from build123d import *

# Parameters (mm, degrees)
SKETCH_1_R      = 1.65
SKETCH_1_R_2    = 5
EXTRUDE_1_DEPTH = 3
FILLET_1_R      = 1


with BuildPart() as part:
    # 草图1 → 凸台-拉伸1 (new body)
    with BuildSketch(Plane.XY):
        with BuildLine():
            Line((-5.5, 2.397915762), (-8, -79.435617584))
            ThreePointArc((-8, -79.435617584), (0, -112.5), (8, -79.435617584))
            Line((8, -79.435617584), (5.5, 2.397915762))
            ThreePointArc((5.5, 2.397915762), (0, 6), (-5.5, 2.397915762))
        make_face()
        Circle(SKETCH_1_R, mode=Mode.SUBTRACT)
        with Locations((0, -95)):
            Circle(SKETCH_1_R_2, mode=Mode.SUBTRACT)
        with BuildLine():
            Line((-3.203324226, -2.80246125), (-3.504023082, -12.645361196))
            Line((-3.504023082, -12.645361196), (3.713679897, -12.645361196))
            Line((3.713679897, -12.645361196), (3.40536458, -2.553148492))
            ThreePointArc((3.40536458, -2.553148492), (0.16045027, -4.253155401), (-3.203324226, -2.80246125))
        make_face(mode=Mode.SUBTRACT)
        Polygon((-3.570265581, -14.813704302), (-3.957626018, -27.493333612), (4.167282834, -27.493333612), (3.779922396, -14.813704302), align=None, mode=Mode.SUBTRACT)
        Polygon((-4.048518432, -30.468552565), (4.258175248, -30.468552565), (4.818203506, -48.800189025), (-4.60854669, -48.800189025), align=None, mode=Mode.SUBTRACT)
        with BuildLine():
            Line((-4.696319338, -51.673287395), (-5.408181825, -74.974976421))
            ThreePointArc((-5.408181825, -74.974976421), (0.132605518, -74.257955362), (5.66377239, -75.045760292))
            Line((5.66377239, -75.045760292), (4.949747468, -51.673287395))
            Line((4.949747468, -51.673287395), (-4.696319338, -51.673287395))
        make_face(mode=Mode.SUBTRACT)
        with BuildLine():
            Line((0, -81), (0, -88))
            ThreePointArc((0, -88), (2.096194278, -88.321229937), (3.999999882, -89.255437272))
            Line((3.999999882, -89.255437272), (7.999999765, -83.510874543))
            ThreePointArc((7.999999765, -83.510874543), (4.192388556, -81.642459875), (0, -81))
        make_face(mode=Mode.SUBTRACT)
        with BuildLine():
            Line((9.899494937, -85.100505063), (4.949747468, -90.050252532))
            ThreePointArc((4.949747468, -90.050252532), (6.20483679, -91.759629587), (6.890446302, -93.766407781))
            Line((6.890446302, -93.766407781), (13.780892604, -92.532815563))
            ThreePointArc((13.780892604, -92.532815563), (12.40967358, -88.519259175), (9.899494937, -85.100505063))
        make_face(mode=Mode.SUBTRACT)
        with BuildLine():
            Line((14, -95), (7, -95))
            ThreePointArc((7, -95), (6.678770063, -97.096194278), (5.744562728, -98.999999882))
            Line((5.744562728, -98.999999882), (11.489125457, -102.999999765))
            ThreePointArc((11.489125457, -102.999999765), (13.357540125, -99.192388556), (14, -95))
        make_face(mode=Mode.SUBTRACT)
        with BuildLine():
            Line((9.899494937, -104.899494937), (4.949747468, -99.949747468))
            ThreePointArc((4.949747468, -99.949747468), (3.240370413, -101.20483679), (1.233592219, -101.890446302))
            Line((1.233592219, -101.890446302), (2.467184437, -108.780892604))
            ThreePointArc((2.467184437, -108.780892604), (6.480740825, -107.40967358), (9.899494937, -104.899494937))
        make_face(mode=Mode.SUBTRACT)
        with BuildLine():
            Line((0, -109), (0, -102))
            ThreePointArc((0, -102), (-2.096194278, -101.678770063), (-3.999999882, -100.744562728))
            Line((-3.999999882, -100.744562728), (-7.999999765, -106.489125457))
            ThreePointArc((-7.999999765, -106.489125457), (-4.192388556, -108.357540125), (0, -109))
        make_face(mode=Mode.SUBTRACT)
        with BuildLine():
            Line((-9.899494937, -104.899494937), (-4.949747468, -99.949747468))
            ThreePointArc((-4.949747468, -99.949747468), (-6.20483679, -98.240370413), (-6.890446302, -96.233592219))
            Line((-6.890446302, -96.233592219), (-13.780892604, -97.467184437))
            ThreePointArc((-13.780892604, -97.467184437), (-12.40967358, -101.480740825), (-9.899494937, -104.899494937))
        make_face(mode=Mode.SUBTRACT)
        with BuildLine():
            Line((-14, -95), (-7, -95))
            ThreePointArc((-7, -95), (-6.678770063, -92.903805722), (-5.744562728, -91.000000118))
            Line((-5.744562728, -91.000000118), (-11.489125457, -87.000000235))
            ThreePointArc((-11.489125457, -87.000000235), (-13.357540125, -90.807611444), (-14, -95))
        make_face(mode=Mode.SUBTRACT)
        with BuildLine():
            Line((-9.899494937, -85.100505063), (-4.949747468, -90.050252532))
            ThreePointArc((-4.949747468, -90.050252532), (-3.240370413, -88.79516321), (-1.233592219, -88.109553698))
            Line((-1.233592219, -88.109553698), (-2.467184437, -81.219107396))
            ThreePointArc((-2.467184437, -81.219107396), (-6.480740825, -82.59032642), (-9.899494937, -85.100505063))
        make_face(mode=Mode.SUBTRACT)
    extrude(amount=EXTRUDE_1_DEPTH)

    # 圆角1
    fillet_1_edges = [part.edges().sort_by_distance(p)[0] for p in [
        (3.40536458, -2.553148492, 1.5),
        (-3.203324226, -2.80246125, 1.5),
        (-3.504023082, -12.645361196, 1.5),
        (3.713679897, -12.645361196, 1.5),
        (-5.408181825, -74.974976421, 1.5),
        (5.66377239, -75.045760292, 1.5),
        (4.949747468, -51.673287395, 1.5),
        (-4.696319338, -51.673287395, 1.5),
        (3.779922396, -14.813704302, 1.5),
        (-3.570265581, -14.813704302, 1.5),
        (-3.957626018, -27.493333612, 1.5),
        (4.167282834, -27.493333612, 1.5),
        (-4.048518432, -30.468552565, 1.5),
        (-4.60854669, -48.800189025, 1.5),
        (4.818203506, -48.800189025, 1.5),
        (4.258175248, -30.468552565, 1.5),
    ]]
    fillet(fillet_1_edges, radius=FILLET_1_R)


solid = part.part
Work out the finished part from the listing and answer in its coordinate system (mm). Coordinates: 2 decimals unless noted, no trailing zeros. Order: outer loops, then holes, each group sorted by start corner. A loop starts at its lowest first (then second) coordinate and runs counter-clockwise, first axis right, second up. Notation, with made-up numbers: (46, 66.25) - (59, 66.25) arc R22 cw to (59, 100.25) - close; hole circle Ø1 at (-22.5, 10). An arc over 180 degrees is marked (long way). Put each result on its own line as item: value. Start each with the question number.
1) Find section A-A (y = -70). Give the vertices of the cut face in (x, z), plus the area to 3 significant figures.
2) Find section C-C (x = 15.5). Give the vertices of the cut face in (y, z).
3) Flat-ended cylindrical pins translate along their axes: pin 1 (8 mm diameter, centred on x = -9.5, y = -20.5, fed in from +Z); pin 2 (1.5 mm diameter, centred on y = -64.5, z = 0.5, fed in from +X); pin 3 (1.5 mm diameter, centred on x = 11, z = 1.5, fed in from -Y); pin 4 (1 mm diameter, centred on x = -1, z = 2, fed in from +Y). Find the tip coordinate at first contact, or state that the pin passes through.
4) Find section D-D (z = 2.05). State how many separate pieces and enclosed holes the cut face has, plus the area to 3 significant figures.
5) Find the intervals of material crossed by line 1 (X direction, y = -86, z = 1.1); line 2 (X direction, y = -67.5, z = 0.2); line 3 (X direction, y = -19, z = 2), in increasing order. Write a range as from..to.
6) Find section B-B (y = 0). Give the vertices of the cut face in (x, z).
Results list:
1. outline: (-7.71, 0) - (-5.26, 0) - (-5.26, 3) - (-7.71, 3) - close; (5.51, 0) - (7.71, 0) - (7.71, 3) - (5.51, 3) - close
1. area: 14.0 mm^2
2. outline: (-103.12, 0) - (-86.88, 0) - (-86.88, 3) - (-103.12, 3) - close
3. pin 1: stops at z = 3
3. pin 2: stops at x = 7.57
3. pin 3: stops at y = -109.18
3. pin 4: stops at y = 5.98
4. separate pieces: 1
4. enclosed holes: 14
4. area: 1,080 mm^2
5. line 1: x = -15.01..-9, -1.61..0, 6.27..9, 10.72..15.01
5. line 2: x = -7.64..-5.18, 5.43..7.64
5. line 3: x = -6.15..-3.7, 3.91..6.15
6. outline: (-5.57, 0) - (-1.65, 0) - (-1.65, 3) - (-5.57, 3) - close; (1.65, 0) - (5.57, 0) - (5.57, 3) - (1.65, 3) - close
